```python
from build123d import *

# Parameters (mm, degrees)
DODANIE_WYCI_GNI_CIE1_DEPTH = 12
SZKIC3_R                    = 2
WYTNIJ_WYCI_GNI_CIE1_DEPTH  = 12
SZKIC6_R                    = 4
WYTNIJ_WYCI_GNI_CIE2_DEPTH  = 12
SZKIC7_R                    = 3
WYTNIJ_WYCI_GNI_CIE3_DEPTH  = 14.5
SZKIC9_R                    = 2.5
WYTNIJ_WYCI_GNI_CIE5_DEPTH  = 13


with BuildPart() as part:
    # Szkic1 → Obrót1 (revolve)
    with BuildSketch(Plane(origin=(0, 0, 0), x_dir=(1, 0, 0), z_dir=(0, 1, 0))):
        Polygon((28.285714286, 0), (40.785714286, 0), (40.785714286, 7.5), (60.785714286, 7.5), (60.785714286, 10.5), (56.785714286, 10.5), (56.785714286, 12), (53.785714286, 12), (53.785714286, 10), (28.285714286, 10), align=None)
    revolve(axis=Axis((28.285714286, 0, 0), (1, 0, 0)))

    # Szkic2 → Dodanie-wyciągnięcie1 (add)
    with BuildSketch(Plane.ZY.offset(-28.285714286)):
        with BuildLine():
            Line((0, -10), (0, 10))
            ThreePointArc((0, 10), (10, 0), (0, -10))
        make_face()
    extrude(amount=DODANIE_WYCI_GNI_CIE1_DEPTH)

    # Szkic3 → Wytnij-wyciągnięcie1 (cut)
    with BuildSketch(Plane.XY):
        with Locations((22.285714286, 4.75)):
            Circle(SZKIC3_R)
        with Locations((22.285714286, -4.75)):
            Circle(SZKIC3_R)
    extrude(amount=WYTNIJ_WYCI_GNI_CIE1_DEPTH, mode=Mode.SUBTRACT)

    # Szkic6 → Wytnij-wyciągnięcie2 (cut)
    with BuildSketch(Plane(origin=(0, 0, 4.5), x_dir=(-1, 0, 0), z_dir=(0, 0, -1))):
        with Locations((-22.285714286, -4.75)):
            Circle(SZKIC6_R)
    extrude(amount=-WYTNIJ_WYCI_GNI_CIE2_DEPTH, mode=Mode.SUBTRACT)

    # Szkic7 → Wytnij-wyciągnięcie3 (cut)
    with BuildSketch(Plane(origin=(40.785714286, 0, 0), x_dir=(0, 0, -1), z_dir=(1, 0, 0))):
        Circle(SZKIC7_R)
    extrude(amount=-WYTNIJ_WYCI_GNI_CIE3_DEPTH, mode=Mode.SUBTRACT)

    # Szkic9 → Wytnij-wyciągnięcie5 (cut, through all)
    with BuildSketch(Plane.XY):
        with Locations((28.285714286, 0)):
            Circle(SZKIC9_R)
    extrude(amount=-WYTNIJ_WYCI_GNI_CIE5_DEPTH, mode=Mode.SUBTRACT)


solid = part.part
```
Design review of the part built by this model. Coordinates are the model's own, in mm. A direction names the side the tool comes from. Give positions to 0.01 mm unless a question says otherwise; leave off trailing zeros. Order: outer loops, then holes, each group sorted by start corner. A loop starts at its lowest first (then second) coordinate and runs counter-clockwise, first axis right, second up. Notation, with made-up numbers: M 1,89 L 13,89 A14 ccw 13,106 Z; hole C 21,-38.75 d5. An arc over 180 degrees is marked long. One line per question, with ' | ' between items. Start each with the question number.
Q1. We need section A-A (y = 0). Write out the cut boundary in (x, z), plus the area to 4 significant figures.
Q2. The part is to be moulded in two halves that separate along Y. For faces 4 (the face through (21, -3, 4.5)), 5 (the face through (28.286, 5, -4)), 6 (the face through (39, 0, 10)), 7 (the face through (40.786, -3.2, -0.1)), say which applies: +Y half, -Y half, draft (parallel to the pull), parting line (faces both ways), or undercut.
Q3. For L1, parallel to Z at x = 37, y = 0; L2, parallel to Y at x = 55.25, z = 0; L3, parallel to X at y = -4.75, z = 7.8, list the stretches that pass through material, from the lowest coordinate up. Write a range as [from, to].
Q4. Machinability: for faces 1 (the face through (34, 0, 3)), 2 (the face through (26.286, 0, 1)), 3 (the face through (30.785, -0.055, -5.771)), which of the approach directions +Z, -Z, +X, -X, +Y, -Y give a long, thin tool a straight path to every point of the face, cutting with its end or side? Answer none if there is none.
Q5. For pin 1 Ø4 at (y, z) = (8, -3) entering from -X; pin 2 Ø4.5 at (x, y) = (22.29, -4.75) entering from -Z; pin 3 Ø1.5 at (x, z) = (44.5, -8) entering from -Y; pin 4 Ø3 at (x, z) = (26.5, -4.5) entering from -Y, all flat-tipped, find the tip position at first contact; note any pin that passes through.
Q6. We need section C-C (z = -8.75). Write out the cut boundary in (x, y), plus the area to 3 significant figures.
Q7. We need section D-D (z = 6). Write out the cut boundary in (x, y), plus the area to 3 significant figures.
Q8. We need section B-B (x = 43.5). Write out the cut boundary in (y, z).
Returned:
1) outline: M 16.29,0 L 26.29,0 L 26.29,3 L 40.79,3 L 40.79,7.5 L 60.79,7.5 L 60.79,10.5 L 56.79,10.5 L 56.79,12 L 53.79,12 L 53.79,10 L 16.29,10 Z; M 30.79,-10 L 53.79,-10 L 53.79,-12 L 56.79,-12 L 56.79,-10.5 L 60.79,-10.5 L 60.79,-7.5 L 40.79,-7.5 L 40.79,-3 L 30.79,-3 Z | area: 387.5 mm2
2) face 4: undercut | face 5: draft | face 6: parting line | face 7: undercut
3) L1: [-10, -3], [3, 10] | L2: [-12, -7.5], [7.5, 12] | L3: [16.29, 18.29], [26.29, 60.79]
4) face 1: +X | face 2: -Z, +X | face 3: -Z, -X
5) pin 1: x = 28.29 | pin 2: z = 0 | pin 3: y = -6.89 | pin 4: through
6) outline: M 28.29,-4.84 L 53.79,-4.84 L 53.79,-8.21 L 56.79,-8.21 L 56.79,-5.8 L 60.79,-5.8 L 60.79,5.8 L 56.79,5.8 L 56.79,8.21 L 53.79,8.21 L 53.79,4.84 L 28.29,4.84 L 28.29,2.5 A2.5 cw 28.29,-2.5 Z | area: 333 mm2
7) outline: M 16.29,-8 L 19.95,-8 A4 cw long 24.62,-8 L 53.79,-8 L 53.79,-10.39 L 56.79,-10.39 L 56.79,-8.62 L 60.79,-8.62 L 60.79,-4.5 L 40.79,-4.5 L 40.79,4.5 L 60.79,4.5 L 60.79,8.62 L 56.79,8.62 L 56.79,10.39 L 53.79,10.39 L 53.79,8 L 16.29,8 Z; hole C 22.29,4.75 d4 | area: 491 mm2
8) outline: C 0,0 d20; hole C 0,0 d15
